Input: part model. Units: mm. Frame: model coordinates. Coordinates: 2 decimals unless noted, no trailing zeros. Write each loop counter-clockwise with the first axis right and the second up, starting at its lowest first coordinate (ties: lowest second). Pieces come first, ordered by that corner, then holes. Notation, with made-up numbers: (-23, 68.5) - (32, 68.5) arc R19 cw to (32, 99.5) - close; hole circle Ø1 at (15.5, 10.5). An arc over 180 degrees is marked (long way). One line per question, with ' | ' between items. Start each with the question number.
1) Section query C-C on x = 31. Return loops of the section in (y, z) (3 decimals), and give its area (3 significant figures).
2) Line query: line 1 (Y direction, x = 0, z = 1.4) (3 decimals); line 2 (X direction, y = 108.5, z = 1.85); line 3 (X direction, y = 98, z = 1.55). Output: solid intervals per line, ascending.
3) Section query A-A on x = 0. Return loops of the section in (y, z) (3 decimals), and give its area (3 significant figures).
4) Section query D-D on y = 122.5. Return loops of the section in (x, z) (3 decimals).
5) First-contact query: P1, Ø1.5, axis at y = 20, z = 2.5, coming from the +X side; P2, Ø1.6, axis at y = 45.5, z = 2.5, coming from the -X side. Flat tips, straight axial feed; report the tip coordinate or a pass-through.
6) Section query B-B on z = 0.85. Return loops of the section in (x, y) (3 decimals).
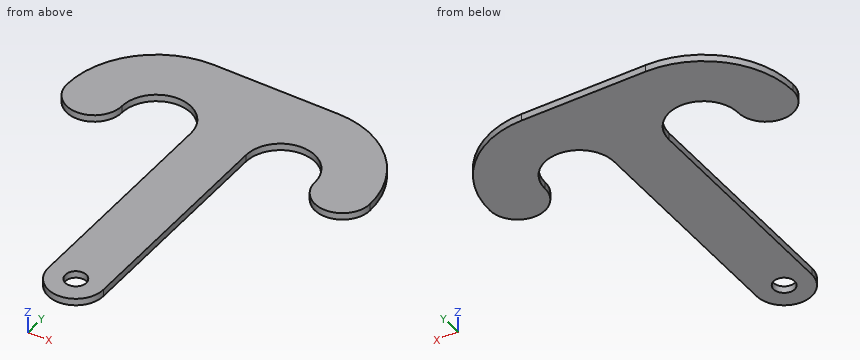
```python
from build123d import *

# Parameters (mm, degrees)
SKETCH1_R           = 4.826
BOSS_EXTRUDE2_DEPTH = 3.175


with BuildPart() as part:
    # Sketch1 → Boss-Extrude2 (new body)
    with BuildSketch(Plane.XY):
        with BuildLine():
            Line((12.7, 0), (12.7, 101.6))
            ThreePointArc((12.7, 101.6), (28.575, 117.475), (44.45, 101.6))
            ThreePointArc((44.45, 101.6), (57.15, 88.9), (69.85, 101.6))
            ThreePointArc((69.85, 101.6), (57.760832393, 130.785832393), (28.575, 142.875))
            Line((28.575, 142.875), (-28.575, 142.875))
            ThreePointArc((-28.575, 142.875), (-57.760832393, 130.785832393), (-69.85, 101.6))
            ThreePointArc((-69.85, 101.6), (-57.15, 88.9), (-44.45, 101.6))
            ThreePointArc((-44.45, 101.6), (-28.575, 117.475), (-12.7, 101.6))
            Line((-12.7, 101.6), (-12.7, 0))
            ThreePointArc((-12.7, 0), (0, -12.7), (12.7, 0))
        make_face()
        Circle(SKETCH1_R, mode=Mode.SUBTRACT)
    extrude(amount=BOSS_EXTRUDE2_DEPTH)


solid = part.part
```
Answer key:
1) outline: (117.289, 0) - (142.804, 0) - (142.804, 3.175) - (117.289, 3.175) - close | area: 81.0 mm²
2) line 1: -12.7 to -4.826, 4.826 to 142.875 | line 2: -69.27 to -42.87, -14.28 to 14.28, 42.87 to 69.27 | line 3: -69.33 to -44.97, -12.7 to 12.7, 44.97 to 69.33
3) outline: (-12.7, 0) - (-4.826, 0) - (-4.826, 3.175) - (-12.7, 3.175) - close; (4.826, 0) - (142.875, 0) - (142.875, 3.175) - (4.826, 3.175) - close | area: 463 mm²
4) outline: (-64.167, 0) - (64.167, 0) - (64.167, 3.175) - (-64.167, 3.175) - close
5) P1: x = 12.7 | P2: x = -12.7
6) outline: (-69.85, 101.6) arc R12.7 ccw to (-44.45, 101.6) arc R15.875 cw to (-12.7, 101.6) - (-12.7, 0) arc R12.7 ccw to (12.7, 0) - (12.7, 101.6) arc R15.875 cw to (44.45, 101.6) arc R12.7 ccw to (69.85, 101.6) arc R41.275 ccw to (28.575, 142.875) - (-28.575, 142.875) arc R41.275 ccw to start; hole circle Ø9.652 at (0, 0)
